Study the drawing (mm; zero at the part's minimum x, y, z) and answer. A direction names the side the tool comes from. Round coordinates to 2 decimals unless told otherwise and drop trailing zeros. Order: outer loops, then holes, each group sorted by start corner. A loop starts at its lowest first (then second) coordinate and runs counter-clockwise, first axis right, second up. Notation, with made-up numbers: (10.25, -27) - (67.25, -27) arc R23 cw to (67.25, -8) - close; hole circle Ø10 at (73.5, 81). An arc over 180 degrees is marked (long way). Put each result on its own line as item: value.
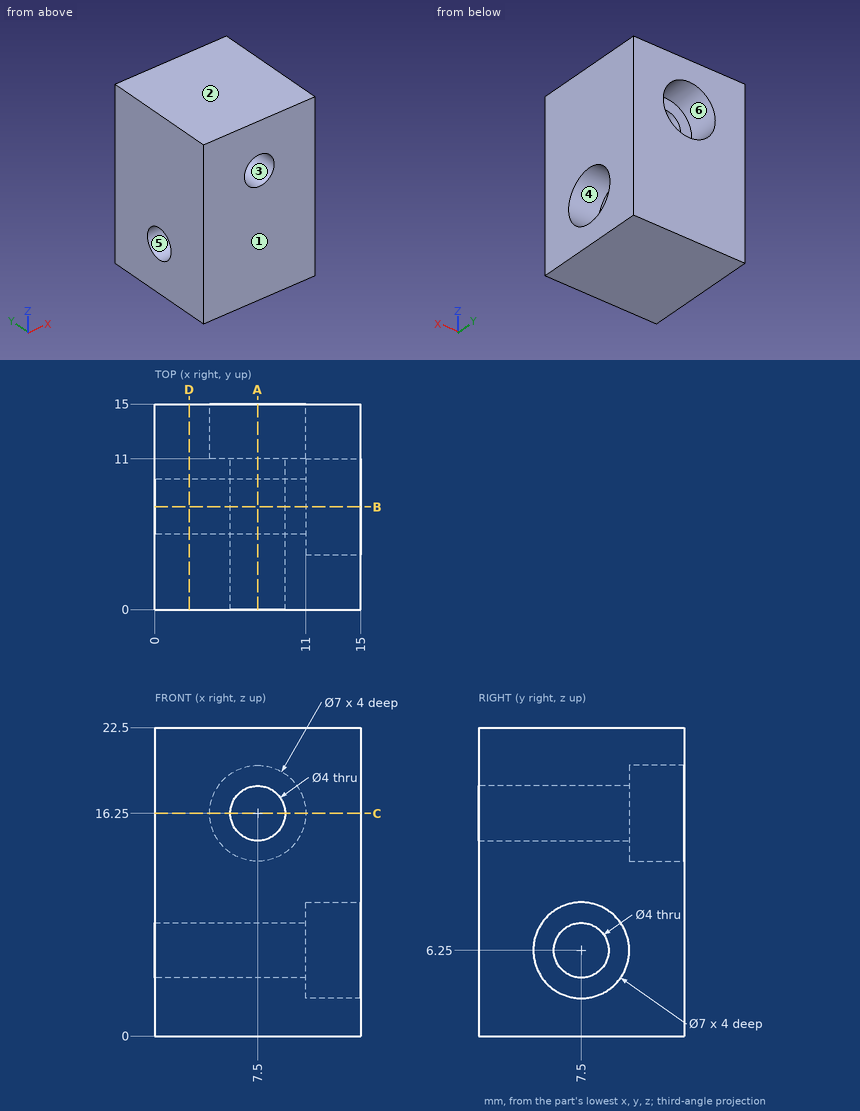
1) For a pull along Z with two mould halves and no side action, classify the marked faces 1, 2 and 3 as pulls with the +Z half, pulls with the -Z half, needs draft (parallel to the pull), parting line crosses it, or undercut.
Findings below:
face 1: needs draft
face 2: pulls with the +Z half
face 3: undercut
2) For the marked faces 4, 5 and 6, determine the directions among +Z, -Z, +X, -X, +Y, -Y from which every point of the face is accessible in a straight line to the end or side of a thin tool.
Findings below:
face 4: +X
face 5: +X, -X
face 6: +Y
3) Given pin 1 Ø5 at (x, y) = (12, 11.5) entering from -Z; pin 2 Ø6.5 at (x, z) = (7.5, 16.25) entering from +Y; pin 3 Ø2 at (y, z) = (7.5, 5.5) entering from +X, each flat-ended and moving along its own axis, determine where each tip first touches the part or whether it passes through.
Findings below:
pin 1: stops at z = 0
pin 2: stops at y = 11
pin 3: passes through
4) A cutting plane is placed at B-B on y = 7.5. Write down the section's boundary in (x, z), then the cut area to 3 significant figures.
Findings below:
outline: (0, 0) - (15, 0) - (15, 2.75) - (11, 2.75) - (11, 4.25) - (0, 4.25) - close; (0, 8.25) - (11, 8.25) - (11, 9.75) - (15, 9.75) - (15, 22.5) - (0, 22.5) - close; hole circle Ø4 at (7.5, 16.25)
area: 253 mm2
5) A cutting plane is placed at D-D on x = 2.5. Write down the section's boundary in (y, z), then the cut area to 3 significant figures.
Findings below:
outline: (0, 0) - (15, 0) - (15, 22.5) - (0, 22.5) - close; hole circle Ø4 at (7.5, 6.25)
area: 325 mm2
6) A cutting plane is placed at C-C on z = 16.25. Write down the section's boundary in (x, y).
Findings below:
outline: (0, 0) - (5.5, 0) - (5.5, 11) - (4, 11) - (4, 15) - (0, 15) - close; (9.5, 0) - (15, 0) - (15, 15) - (11, 15) - (11, 11) - (9.5, 11) - close
7) Straight lines are drawn through the part: L1, parallel to Y at x = 4.75, z = 6.25; L2, parallel to Y at x = 14.2, z = 6.25; L3, parallel to Z at x = 3, y = 6.75. For each, find the intervals that lie inside material, in ascending order. Write a range as from..to.
Findings below:
L1: y = 0..5.5, 9.5..15
L2: y = 0..4, 11..15
L3: z = 0..4.4, 8.1..22.5
8) A cutting plane is placed at A-A on x = 7.5. Write down the section's boundary in (y, z), then the cut area to 3 significant figures.
Findings below:
outline: (0, 0) - (15, 0) - (15, 12.75) - (11, 12.75) - (11, 14.25) - (0, 14.25) - close; (0, 18.25) - (11, 18.25) - (11, 19.75) - (15, 19.75) - (15, 22.5) - (0, 22.5) - close; hole circle Ø4 at (7.5, 6.25)
area: 253 mm2
